Design review of the part built by this model. Coordinates are the model's own, in mm. Face numbers are marked on the shaded views. A direction names the side the tool comes from. Give positions to 0.01 mm unless a question says otherwise; leave off trailing zeros. Order: outer loops, then holes, each group sorted by start corner. A loop starts at its lowest first (then second) coordinate and runs counter-clockwise, first axis right, second up.
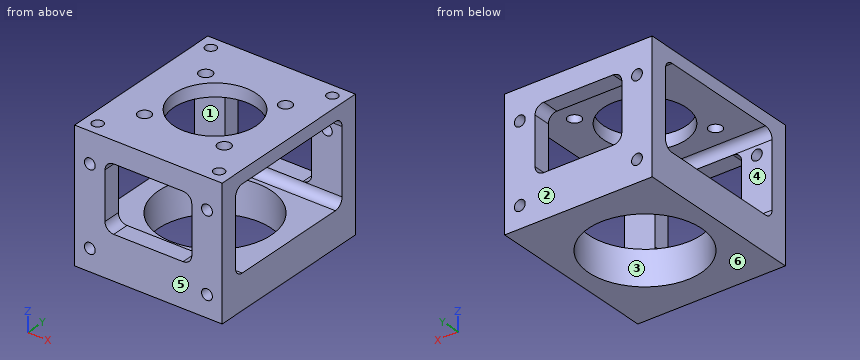
```python
from build123d import *

# Parameters (mm, degrees)
SKETCH_1_W                = 34
SKETCH_1_H                = 40
SKETCH_1_R                = 9.5
EXTRUDE_1_DEPTH           = 30
SKETCH_3_W                = 19
SKETCH_3_H                = 32
CUT_EXTRUDE_1_DEPTH       = 61.464865831
FILLET_3_R                = 2
HOLE_WIZARD_M3_2_D        = 2.5
HOLE_WIZARD_M3_2_DEPTH    = 4
HOLE_WIZARD_M3_2_TIP      = 0.751075774
HOLE_WIZARD_M3_4_D        = 2.5
HOLE_WIZARD_M3_4_DEPTH    = 4
HOLE_WIZARD_M3_4_TIP      = 0.751075774
SKETCH_18_W               = 20
SKETCH_18_H               = 15
CUT_EXTRUDE_8_DEPTH       = 61.464865831
SKETCH_12_R               = 13
CUT_EXTRUDE_6_DEPTH       = 8
HOLE_WIZARD_3_0_3_1_D     = 3
HOLE_WIZARD_3_0_3_1_DEPTH = 3
FILLET_7_R                = 2
HOLE_WIZARD_M3_3_D        = 2.5
HOLE_WIZARD_M3_3_DEPTH    = 4
HOLE_WIZARD_M3_3_TIP      = 0.751075774


with BuildPart() as part:
    # 草图1 → 凸台-拉伸1 (new body)
    with BuildSketch(Plane.XY):
        with Locations((17, 20)):
            Rectangle(SKETCH_1_W, SKETCH_1_H)
        with Locations((17, 20)):
            Circle(SKETCH_1_R, mode=Mode.SUBTRACT)
    extrude(amount=EXTRUDE_1_DEPTH)

    # 草图3 → 切除-拉伸1 (cut, through all)
    with BuildSketch(Plane.ZY):
        with Locations((17.5, 20)):
            Rectangle(SKETCH_3_W, SKETCH_3_H)
    extrude(amount=-CUT_EXTRUDE_1_DEPTH, mode=Mode.SUBTRACT)

    # 圆角3
    fillet_3_edges = [part.edges().sort_by_distance(p)[0] for p in [
        (17, 36, 27),
        (17, 4, 27),
        (17, 4, 8),
        (17, 36, 8),
    ]]
    fillet(fillet_3_edges, radius=FILLET_3_R)

    # M3 螺纹孔2
    with Locations(Plane(origin=(3.5, 40, 5), x_dir=(0, 0, 1), z_dir=(0, 1, 0))):
        with Locations((0, 0), (0, 27), (18, 27), (18, 0)):
            Hole(HOLE_WIZARD_M3_2_D / 2, depth=HOLE_WIZARD_M3_2_DEPTH)
            with Locations((0, 0, -(HOLE_WIZARD_M3_2_DEPTH + HOLE_WIZARD_M3_2_TIP / 2))):  # 118° drill point
                Cone(0, HOLE_WIZARD_M3_2_D / 2, HOLE_WIZARD_M3_2_TIP, mode=Mode.SUBTRACT)

    # M3 螺纹孔4
    with Locations(Plane(origin=(3.5, 0, 5), x_dir=(0, 0, -1), z_dir=(0, -1, 0))):
        with Locations((0, 0), (-18, 0), (-18, 27), (0, 27)):
            Hole(HOLE_WIZARD_M3_4_D / 2, depth=HOLE_WIZARD_M3_4_DEPTH)
            with Locations((0, 0, -(HOLE_WIZARD_M3_4_DEPTH + HOLE_WIZARD_M3_4_TIP / 2))):  # 118° drill point
                Cone(0, HOLE_WIZARD_M3_4_D / 2, HOLE_WIZARD_M3_4_TIP, mode=Mode.SUBTRACT)

    # 草图18 → 切除-拉伸8 (cut, through all)
    with BuildSketch(Plane(origin=(0, 40, 0), x_dir=(1, 0, 0), z_dir=(0, 1, 0))):
        with Locations((17, -17.5)):
            Rectangle(SKETCH_18_W, SKETCH_18_H)
    extrude(amount=-CUT_EXTRUDE_8_DEPTH, mode=Mode.SUBTRACT)

    # 草图12 → 切除-拉伸6 (cut)
    with BuildSketch(Plane(origin=(0, 0, 0), x_dir=(-1, 0, 0), z_dir=(0, 0, -1))):
        with Locations((-17, 20)):
            Circle(SKETCH_12_R)
    extrude(amount=-CUT_EXTRUDE_6_DEPTH, mode=Mode.SUBTRACT)

    # Ø3.0 (3) 直径孔1
    with Locations(Plane(origin=(7.807611845, 29.192388155, 30), x_dir=(1, 0, 0), z_dir=(0, 0, 1))):
        with Locations((0, 0), (18.38477631, 0), (18.38477631, -18.38477631), (0, -18.38477631)):
            Hole(HOLE_WIZARD_3_0_3_1_D / 2, depth=HOLE_WIZARD_3_0_3_1_DEPTH)

    # 圆角7
    fillet_7_edges = [part.edges().sort_by_distance(p)[0] for p in [
        (27, 38, 25),
        (27, 2, 25),
        (27, 2, 10),
        (27, 38, 10),
        (7, 2, 25),
        (7, 38, 25),
        (7, 38, 10),
        (7, 2, 10),
    ]]
    fillet(fillet_7_edges, radius=FILLET_7_R)

    # M3 螺纹孔3
    with Locations(Plane(origin=(3, 37, 30), x_dir=(1, 0, 0), z_dir=(0, 0, 1))):
        with Locations((0, 0), (28, 0), (28, -34), (0, -34)):
            Hole(HOLE_WIZARD_M3_3_D / 2, depth=HOLE_WIZARD_M3_3_DEPTH)
            with Locations((0, 0, -(HOLE_WIZARD_M3_3_DEPTH + HOLE_WIZARD_M3_3_TIP / 2))):  # 118° drill point
                Cone(0, HOLE_WIZARD_M3_3_D / 2, HOLE_WIZARD_M3_3_TIP, mode=Mode.SUBTRACT)


solid = part.part
```
1. Take a section at C-C (x = 13). State the section outline as (y, z) points, then the cut area to 3 significant figures.
Recorded:
outline: (0, 0) - (7.63, 0) - (7.63, 8) - (6, 8) arc R2 cw to (4, 10) - (0, 10) - close; (0, 25) - (4, 25) arc R2 cw to (6, 27) - (11.38, 27) - (11.38, 30) - (0, 30) - close; (28.62, 27) - (34, 27) arc R2 cw to (36, 25) - (40, 25) - (40, 30) - (28.62, 30) - close; (32.37, 0) - (40, 0) - (40, 10) - (36, 10) arc R2 cw to (34, 8) - (32.37, 8) - close
area: 226 mm2
2. Machinability: for the marked faces 1, 2 and 3, which of the approach directions +Z, -Z, +X, -X, +Y, -Y give a long, thin tool a straight path to every point of the face, cutting with its end or side? Answer none if there is none.
Recorded:
face 1: +X, -X
face 2: +Z, -Z, +X, -X, +Y
face 3: -Z
3. For line 1 along Y through (x, z) = (3, 28.15); line 2 along X through (y, z) = (2.4, 5); line 3 along Z through (x, y) = (10.5, 6.5), list the stretches that pass through material, from the lowest coordinate up.
Recorded:
line 1: y = 0 to 1.75, 4.25 to 35.75, 38.25 to 40
line 2: x = 0 to 2.25, 4.75 to 29.25, 31.75 to 34
line 3: z = 0 to 8, 27 to 30
4. Take a section at D-D (z = 9.5). State the section outline as (x, y) points.
Recorded:
outline: (0, 0) - (34, 0) - (34, 4.06) - (0, 4.06) - close; (0, 35.94) - (34, 35.94) - (34, 40) - (0, 40) - close
5. Take a section at A-A (y = 20). State the section outline as (x, z) points.
Recorded:
outline: (0, 0) - (4, 0) - (4, 8) - (0, 8) - close; (0, 27) - (7.5, 27) - (7.5, 30) - (0, 30) - close; (26.5, 27) - (34, 27) - (34, 30) - (26.5, 30) - close; (30, 0) - (34, 0) - (34, 8) - (30, 8) - close
6. Draft analysis for pull direction Y (two halves, no side actions). For the marked faces 4, 5 and 6, state which applies: pulls with the +Y half, pulls with the -Y half, needs draft (parallel to the pull), parting line crosses it, or undercut.
Recorded:
face 4: undercut
face 5: pulls with the -Y half
face 6: needs draft
7. For pin 1 (2 mm diameter, centred on x = 31, y = 3, fed in from +Z), flat-tipped, find the tip position at first contact; note if it passes through.
Recorded:
pin 1: stops at z = 25.85
8. Take a section at B-B (z = 2). State the section outline as (x, y) points.
Recorded:
outline: (0, 0) - (34, 0) - (34, 40) - (0, 40) - close; hole circle Ø26 at (17, 20)
